Part model, mm, in its own coordinate system. A direction names the side the tool comes from. Round coordinates to 2 decimals unless told otherwise and drop trailing zeros. Write each loop counter-clockwise with the first axis right and the second up, starting at its lowest first coordinate (ties: lowest second). Pieces come first, ordered by that corner, then holes. Notation, with made-up numbers: M 11.5,3 L 31.5,3 A29 cw 31.5,23 Z; hole C 29.5,21.25 d7. An arc over 180 degrees is marked long. Use a Markdown table: item, result. Add a question column.
1) Slice it at B-B on y = 44.45. Write the cut outline in (x, z), plus the area to 3 significant figures.
2) Wall check: probe 1 along Y at (x, z) = (2.5, 12.5) (3 decimals); probe 2 along Z at (x, y) = (1, 36). Give the ranges that are in metal, low to high.
3) Drop a flat-ended pin along its axis: P1, Ø3, axis at y = -1.59, z = -7.94, coming from the +X side. Give the stop position or say it passes through.
4) Slice it at D-D on x = 2.25. Give the number of separate pieces and of enclosed holes in the cut face, plus the area to 3 significant figures.
5) Which spindle directions (+Z, -Z, +X, -X, +Y, -Y) get a long thin tool onto all of the face, cutting with end or side? Do faces 3 (the face through (3, 19, -69.342)), 4 (the face through (0, 17, 1)). Say none if no direction does.
6) Two-plate mould, pull along Y, no slides. Class faces 1 (the face through (3, -38.1, -38)), 2 (the face through (3, -1, -82.55)): released by +Y, released by -Y, zero draft, split by the parting line, or undercut.
7) Slice it at A-A on z = 44.45. Write the cut outline in (x, y).
8) Slice it at C-C on z = 0. Write the cut outline in (x, y) (3 decimals), plus the area to 3 significant figures.
```python
from build123d import *

# Parameters (mm, degrees)
SKETCH1_W                                         = 165.1
SKETCH1_H                                         = 139.7
BOSS_EXTRUDE1_DEPTH                               = 6.604
SKETCH2_R                                         = 7.874
SKETCH2_W                                         = 28.575
SKETCH2_H                                         = 38.1
CUT_EXTRUDE1_DEPTH                                = 7.604
SKETCH3_R                                         = 2.15265
SKETCH3_W                                         = 6.35
SKETCH3_H                                         = 6.604
CUT_EXTRUDE2_DEPTH                                = 7.604
SKETCH4_R                                         = 1.5875
SKETCH4_W                                         = 19.05
SKETCH4_H                                         = 9.525
CUT_EXTRUDE3_DEPTH                                = 7.604
LPATTERN1_COUNT                                   = 3
LPATTERN1_PITCH                                   = 15.875
FILLET1_R                                         = 3.175
SKETCH5_R                                         = 2.15265
SKETCH5_W                                         = 6.604
SKETCH5_H                                         = 6.35
CUT_EXTRUDE4_DEPTH                                = 7.604
CSK_FOR_8_FLAT_HEAD_SOCKET_CAP_SCREW1_D           = 4.3053
CSK_FOR_8_FLAT_HEAD_SOCKET_CAP_SCREW1_CSINK_D     = 9.1186
CSK_FOR_8_FLAT_HEAD_SOCKET_CAP_SCREW1_CSINK_ANGLE = 82
LPATTERN2_COUNT                                   = 2
LPATTERN2_PITCH                                   = 44.45


with BuildPart() as part:
    # Sketch1 → Boss-Extrude1 (new body)
    with BuildSketch(Plane(origin=(0, 0, 0), x_dir=(0, 0, -1), z_dir=(1, 0, 0))):
        Rectangle(SKETCH1_W, SKETCH1_H)
    extrude(amount=BOSS_EXTRUDE1_DEPTH)

    # Sketch2 → Cut-Extrude1 (cut, through all)
    with BuildSketch(Plane(origin=(6.604, 0, 0), x_dir=(0, 0, -1), z_dir=(1, 0, 0))):
        with Locations((50.8, 44.45)):
            Circle(SKETCH2_R)
        with Locations((25.4, 44.45)):
            Circle(SKETCH2_R)
        with Locations((0, 44.45)):
            Circle(SKETCH2_R)
        with Locations((-42.8625, -19.05)):
            Rectangle(SKETCH2_W, SKETCH2_H)
    extrude(amount=-CUT_EXTRUDE1_DEPTH, mode=Mode.SUBTRACT)

    # Sketch3 → Cut-Extrude2 (cut, through all)
    with BuildSketch(Plane(origin=(6.604, 0, 0), x_dir=(0, 0, -1), z_dir=(1, 0, 0))):
        with Locations((-44.45, -50.8)):
            Circle(SKETCH3_R)
        with Locations((44.45, -50.8)):
            Circle(SKETCH3_R)
        with Locations((-34.925, -50.8)):
            Rectangle(SKETCH3_W, SKETCH3_H)
        with Locations((-53.975, -50.8)):
            Rectangle(SKETCH3_W, SKETCH3_H)
        with Locations((53.975, -50.8)):
            Rectangle(SKETCH3_W, SKETCH3_H)
        with Locations((34.925, -50.8)):
            Rectangle(SKETCH3_W, SKETCH3_H)
    extrude(amount=-CUT_EXTRUDE2_DEPTH, mode=Mode.SUBTRACT)

    # Sketch4 → Cut-Extrude3 (cut, through all)
    with BuildSketch(Plane(origin=(6.604, 0, 0), x_dir=(0, 0, -1), z_dir=(1, 0, 0))):
        with Locations((-20.6375, -33.3375)):
            Circle(SKETCH4_R)
        with Locations((7.9375, -33.3375)):
            Circle(SKETCH4_R)
        with Locations((-6.35, -33.3375)):
            Rectangle(SKETCH4_W, SKETCH4_H)
    cut_extrude3 = extrude(amount=-CUT_EXTRUDE3_DEPTH, mode=Mode.SUBTRACT)

    # LPattern1: Cut-Extrude3 ×3
    with Locations(*[(0, i * LPATTERN1_PITCH, 0) for i in range(1, LPATTERN1_COUNT)]):
        add(cut_extrude3, mode=Mode.SUBTRACT)

    # Fillet1
    fillet1_edges = [part.edges().sort_by_distance(p)[0] for p in [
        (3.302, 69.85, 82.55),
        (3.302, 69.85, -82.55),
        (3.302, -69.85, -82.55),
        (3.302, -69.85, 82.55),
    ]]
    fillet(fillet1_edges, radius=FILLET1_R)

    # Sketch5 → Cut-Extrude4 (cut, through all)
    with BuildSketch(Plane(origin=(6.604, 0, 0), x_dir=(0, 0, -1), z_dir=(1, 0, 0))):
        with Locations((72.644, 28.575)):
            Circle(SKETCH5_R)
        with Locations((-72.644, 28.575)):
            Circle(SKETCH5_R)
        with Locations((72.644, 19.05)):
            Rectangle(SKETCH5_W, SKETCH5_H)
        with Locations((72.644, 38.1)):
            Rectangle(SKETCH5_W, SKETCH5_H)
        with Locations((-72.644, 38.1)):
            Rectangle(SKETCH5_W, SKETCH5_H)
        with Locations((-72.644, 19.05)):
            Rectangle(SKETCH5_W, SKETCH5_H)
    extrude(amount=-CUT_EXTRUDE4_DEPTH, mode=Mode.SUBTRACT)

    # CSK for #8 Flat Head Socket Cap Screw1 (through all)
    with Locations(Plane(origin=(6.604, 0, 0), x_dir=(0, 0, -1), z_dir=(1, 0, 0))):
        with Locations((-72.644, 28.575), (-44.45, -50.8), (44.45, -50.8), (72.644, 28.575)):
            CounterSinkHole(CSK_FOR_8_FLAT_HEAD_SOCKET_CAP_SCREW1_D / 2, CSK_FOR_8_FLAT_HEAD_SOCKET_CAP_SCREW1_CSINK_D / 2, counter_sink_angle=CSK_FOR_8_FLAT_HEAD_SOCKET_CAP_SCREW1_CSINK_ANGLE)

    # LPattern2: Cut-Extrude3 ×2
    with Locations(*[(0, 0, -i * LPATTERN2_PITCH) for i in range(1, LPATTERN2_COUNT)]):
        add(cut_extrude3, mode=Mode.SUBTRACT)


solid = part.part
```
Entries:
| question | item | result |
|---|---|---|
| 1 | outline | M 0,-82.55 L 6.6,-82.55 L 6.6,-58.67 L 0,-58.67 Z; M 0,-42.93 L 6.6,-42.93 L 6.6,-33.27 L 0,-33.27 Z; M 0,-17.53 L 6.6,-17.53 L 6.6,-7.87 L 0,-7.87 Z; M 0,7.87 L 6.6,7.87 L 6.6,82.55 L 0,82.55 Z |
| 1 | area | 778 mm^2 |
| 2 | probe 1 | y = -69.85 to -38.1, -28.575 to -22.225, -12.7 to -6.35, 3.175 to 69.85 |
| 2 | probe 2 | z = -82.55 to -75.95, -69.34 to 69.34, 75.95 to 82.55 |
| 3 | P1 | passes through |
| 4 | separate pieces | 1 |
| 4 | enclosed holes | 28 |
| 4 | area | 20,200 mm^2 |
| 5 | face 3 | +X, -X |
| 5 | face 4 | +Z, -Z, -X, +Y, -Y |
| 6 | face 1 | undercut |
| 6 | face 2 | zero draft |
| 7 | outline | M 0,-69.85 L 6.6,-69.85 L 6.6,-55.36 L 3.84,-52.95 L 0,-52.95 Z; M 0,-48.65 L 3.84,-48.65 L 6.6,-46.24 L 6.6,-38.1 L 0,-38.1 Z; M 0,0 L 6.6,0 L 6.6,69.85 L 0,69.85 Z |
| 8 | outline | M 0,-69.85 L 6.604,-69.85 L 6.604,-38.1 L 0,-38.1 Z; M 0,-28.575 L 6.604,-28.575 L 6.604,-22.225 L 0,-22.225 Z; M 0,-12.7 L 6.604,-12.7 L 6.604,-6.35 L 0,-6.35 Z; M 0,3.175 L 6.604,3.175 L 6.604,36.576 L 0,36.576 Z; M 0,52.324 L 6.604,52.324 L 6.604,69.85 L 0,69.85 Z |
| 8 | area | 630 mm^2 |
